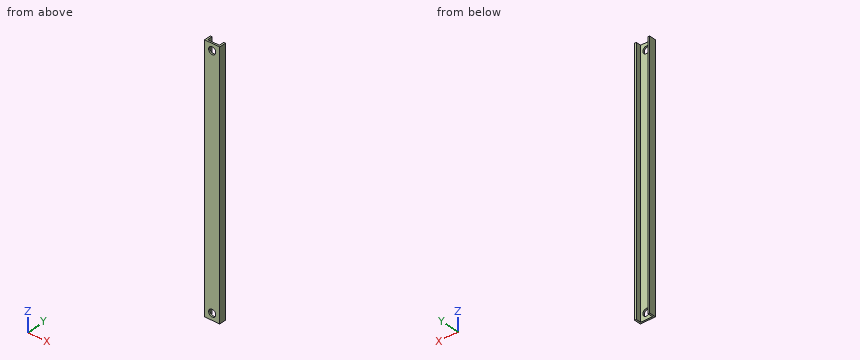
from build123d import *

# Parameters (mm, degrees)
BOSS_EXTRUDE1_DEPTH     = 120.65
F_1_4_CLEARANCE_HOLE1_D = 6.7564


with BuildPart() as part:
    # Sketch2 → Boss-Extrude1 (new, symmetric)
    with BuildSketch(Plane.XY):
        Polygon((-7.14375, 3.175), (-7.14375, -3.175), (7.14375, -3.175), (7.14375, 3.175), (5.55625, 3.175), (5.55625, -1.651), (-5.55625, -1.651), (-5.55625, 3.175), align=None)
    extrude(amount=BOSS_EXTRUDE1_DEPTH, both=True)

    # 1/4 Clearance Hole1 (through all)
    with Locations(Plane(origin=(0, -1.651, 0), x_dir=(-1, 0, 0), z_dir=(0, 1, 0))):
        with Locations((0, -114.3), (0, 114.3)):
            Hole(F_1_4_CLEARANCE_HOLE1_D / 2)


solid = part.part
Work out the finished part from the listing and answer in its coordinate system (mm). Coordinates: 2 decimals unless noted, no trailing zeros. Write each loop counter-clockwise with the first axis right and the second up, starting at its lowest first coordinate (ties: lowest second). Pieces come first, ordered by that corner, then holes.
1. The part is cut by section D-D, the plane z = -14.5. Write down the section's boundary in (x, y) (3 decimals), and give its area (3 significant figures).
Results list:
outline: (-7.144, -3.175) - (7.144, -3.175) - (7.144, 3.175) - (5.556, 3.175) - (5.556, -1.651) - (-5.556, -1.651) - (-5.556, 3.175) - (-7.144, 3.175) - close
area: 37.1 mm2
2. The part is cut by section B-B, the plane y = 2. Write down the section's boundary in (x, z).
Results list:
outline: (-7.14, -120.65) - (-5.56, -120.65) - (-5.56, 120.65) - (-7.14, 120.65) - close; (5.56, -120.65) - (7.14, -120.65) - (7.14, 120.65) - (5.56, 120.65) - close
3. The part is cut by section C-C, the plane x = -0.75. Write down the section's boundary in (y, z) (3 decimals).
Results list:
outline: (-3.175, -120.65) - (-1.651, -120.65) - (-1.651, -117.594) - (-3.175, -117.594) - close; (-3.175, -111.006) - (-1.651, -111.006) - (-1.651, 111.006) - (-3.175, 111.006) - close; (-3.175, 117.594) - (-1.651, 117.594) - (-1.651, 120.65) - (-3.175, 120.65) - close
4. Consider line 1 along Z through (x, y) = (0, -2.5); line 2 along X through (y, z) = (1.5, 87.5); line 3 along Z through (x, y) = (-1, -2.25). Determine where each line is inside the solid, lowest interval first.
Results list:
line 1: z = -120.65 to -117.68, -110.92 to 110.92, 117.68 to 120.65
line 2: x = -7.14 to -5.56, 5.56 to 7.14
line 3: z = -120.65 to -117.53, -111.07 to 111.07, 117.53 to 120.65
5. Flat-ended cylindrical pins translate along their axes: pin 1 (3 mm diameter, centred on x = -3.5, z = -14, fed in from +Y); pin 2 (1 mm diameter, centred on x = -4, y = 0, fed in from +Z). Find the tip coordinate at first contact, or state that the pin passes through.
Results list:
pin 1: stops at y = -1.65
pin 2: passes through
6. The part is cut by section A-A, the plane z = 114.3. Write down the section's boundary in (x, y) (3 decimals), and give its area (3 significant figures).
Results list:
outline: (-7.144, -3.175) - (-3.378, -3.175) - (-3.378, -1.651) - (-5.556, -1.651) - (-5.556, 3.175) - (-7.144, 3.175) - close; (3.378, -3.175) - (7.144, -3.175) - (7.144, 3.175) - (5.556, 3.175) - (5.556, -1.651) - (3.378, -1.651) - close
area: 26.8 mm2
